```python
from build123d import *

# Parameters (mm, degrees)
SKETCH1_W           = 19.05
SKETCH1_H           = 12.7
BOSS_EXTRUDE1_DEPTH = 0.79375
SKETCH2_R           = 0.79375
BOSS_EXTRUDE2_DEPTH = 19.05
CUT_EXTRUDE2_DEPTH  = 20.05


with BuildPart() as part:
    # Sketch1 → Boss-Extrude1 (new body)
    with BuildSketch(Plane(origin=(0, 0, 0), x_dir=(1, 0, 0), z_dir=(0, 1, 0))):
        with Locations((9.525, 6.35)):
            Rectangle(SKETCH1_W, SKETCH1_H)
    extrude(amount=BOSS_EXTRUDE1_DEPTH)

    # Sketch2 → Boss-Extrude2 (add)
    with BuildSketch(Plane(origin=(19.05, 0, 0), x_dir=(0, 0, -1), z_dir=(1, 0, 0))):
        with Locations((13.387407664, 0.396875)):
            Circle(SKETCH2_R)
    extrude(amount=-BOSS_EXTRUDE2_DEPTH)

    # Sketch4 → Cut-Extrude2 (cut, through all)
    with BuildSketch(Plane(origin=(19.05, 0, 0), x_dir=(0, 0, -1), z_dir=(1, 0, 0))):
        Polygon((0, 0.396875), (13.387407664, 0.396875), (13.387407664, 1.190625), (14.181157664, 1.190625), (14.181157664, -0.396875), (0, -0.396875), align=None)
    extrude(amount=-CUT_EXTRUDE2_DEPTH, mode=Mode.SUBTRACT)


solid = part.part
```
The listing builds one solid part. Answer for the finished solid, in the listing's coordinates (mm). A direction names the side the tool comes from. Coordinates: 2 decimals unless noted, no trailing zeros. Loops run counter-clockwise (first coordinate to the right, second up) from the corner with the lowest first, then second, coordinate; pieces in that order, holes last. Notation, with made-up numbers: (-3, 2.25) -> (55, 2.25) arc R21 cw to (55, 17.25) -> close; hole circle Ø10 at (36, 0). An arc over 180 degrees is marked (long way). Return JSON: item names as keys, results as strings. Group by question number.
(1) Given pin 1 Ø1 at (x, z) = (7, -2.5) entering from +Y, flat-ended and moving along its own axis, determine where the tip first touches the part or whether it passes through.
(2) A cutting plane is placed at A-A on x = 2.25. Write down the section's boundary in (y, z), and give its area (3 significant figures).
(3) Which of the six approach directions +Z, -Z, +X, -X, +Y, -Y give full straight-line access (tool end or side, diameter ignored) to faces 1 (the flat face through (10, 0.397, -7)), 2 (the flat face through (9, 0.794, -6))?
(4) A cutting plane is placed at C-C on y = 1. Write down the section's boundary in (x, z).
(5) A cutting plane is placed at B-B on z = -2.25. Write down the section's boundary in (x, y), and give its area (3 significant figures).
(6) Find the intervals of material crossed by probe 1 along Y at (x, z) = (3.75, -12.25); probe 2 along Z at (x, y) = (12.25, 1.1); probe 3 along Z at (x, y) = (6.5, 0.95), in increasing order. Write a range as from..to.
The answers:
{
 "1": {"pin 1": "stops at y = 0.79"},
 "2": {"outline": "(0.4, -13.39) -> (1.19, -13.39) arc R0.79 ccw to (0.79, -12.7) -> (0.79, 0) -> (0.4, 0) -> close", "area": "5.51 mm^2"},
 "3": {"face 1": "+Z, -Z, +X, -X, -Y", "face 2": "+Z, +X, -X, +Y"},
 "4": {"outline": "(0, -13.39) -> (19.05, -13.39) -> (19.05, -12.87) -> (0, -12.87) -> close"},
 "5": {"outline": "(0, 0.4) -> (19.05, 0.4) -> (19.05, 0.79) -> (0, 0.79) -> close", "area": "7.56 mm^2"},
 "6": {"probe 1": "y = 0.4..0.79", "probe 2": "z = -13.39..-13.02", "probe 3": "z = -13.39..-12.82"}
}
